Part print with two shaded views. Sizes in mm from the minimum x, y, z corner. A direction names the side the tool comes from. Coordinates: 2 decimals unless noted, no trailing zeros. Loops run counter-clockwise (first coordinate to the right, second up) from the corner with the lowest first, then second, coordinate; pieces in that order, holes last.
Item 1: Cut at B-B (y = 9.75). List the corners of the cut face in (x, z) (3 decimals), and give its area (3 significant figures).
Item 2: Cut at C-C (x = 21.75). List the corners of the cut face in (y, z), and give its area (4 significant figures).
Item 3: Drill centre lines: line 1 along Z through (x, y) = (21.75, 10.5); line 2 along X through (y, z) = (9.75, 3.25) (3 decimals); line 3 along Y through (x, z) = (27, 7.5). Where is each one in solid material? Low to high.
Item 4: Cut at D-D (x = 38.5). List the corners of the cut face in (y, z), and give its area (3 significant figures).
Item 5: Cut at A-A (z = 4.5). List the corners of the cut face in (x, y) (3 decimals).
Item 6: 3-axis set-ups, long thin cutter, end or side, ignore diameter. For the marked faces 1, 2 and 3: which of +Z, -Z, +X, -X, +Y, -Y reach the whole face in a straight line?
Item 7: Mould opens along Y. For the marked faces 4, 5 and 6 say: released by +Y, released by -Y, zero draft, split by the parting line, or undercut.
Item 8: Flat gauge pins, fed straight in: pin 1 (0.9 mm diameter, centred on y = 14, z = 8.5, fed in from -X); pin 2 (4 mm diameter, centred on x = 5, z = 5.5, fed in from -Y); pin 3 (6 mm diameter, centred on x = 32.625, y = 9.75, fed in from +Z). Where does each tip first touch, or does it go through?
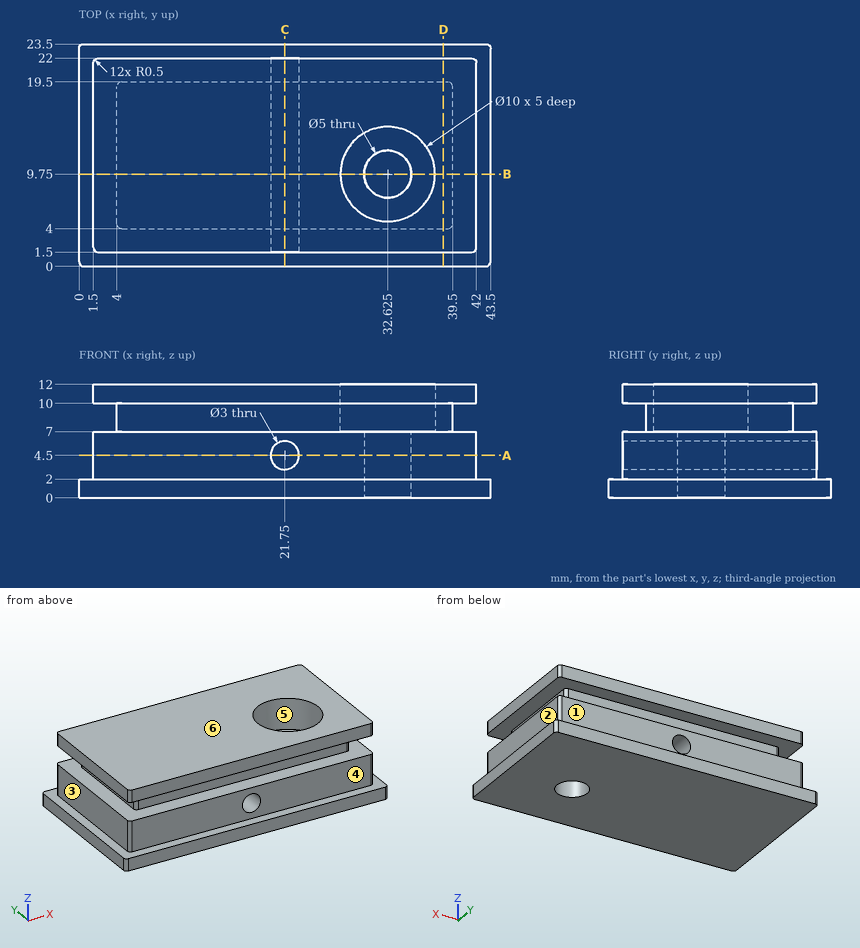
Filled sheet:
1. outline: (0, 0) - (30.125, 0) - (30.125, 7) - (27.625, 7) - (27.625, 12) - (1.5, 12) - (1.5, 10) - (4, 10) - (4, 7) - (1.5, 7) - (1.5, 2) - (0, 2) - close; (35.125, 0) - (43.5, 0) - (43.5, 2) - (42, 2) - (42, 7) - (39.5, 7) - (39.5, 10) - (42, 10) - (42, 12) - (37.625, 12) - (37.625, 7) - (35.125, 7) - close; hole circle Ø3 at (21.75, 4.5)
1. area: 385 mm2
2. outline: (0, 0) - (23.5, 0) - (23.5, 2) - (22, 2) - (22, 3) - (1.5, 3) - (1.5, 2) - (0, 2) - close; (1.5, 6) - (22, 6) - (22, 7) - (19.5, 7) - (19.5, 10) - (22, 10) - (22, 12) - (1.5, 12) - (1.5, 10) - (4, 10) - (4, 7) - (1.5, 7) - close
2. area: 175.5 mm2
3. line 1: z = 0 to 3, 6 to 12
3. line 2: x = 1.5 to 20.921, 22.579 to 30.125, 35.125 to 42
3. line 3: y = 4 to 19.5
4. outline: (0, 0) - (23.5, 0) - (23.5, 2) - (22, 2) - (22, 7) - (19.5, 7) - (19.5, 10) - (22, 10) - (22, 12) - (1.5, 12) - (1.5, 10) - (4, 10) - (4, 7) - (1.5, 7) - (1.5, 2) - (0, 2) - close
4. area: 237 mm2
5. outline: (1.5, 2) arc R0.5 ccw to (2, 1.5) - (20.25, 1.5) - (20.25, 22) - (2, 22) arc R0.5 ccw to (1.5, 21.5) - close; (23.25, 1.5) - (41.5, 1.5) arc R0.5 ccw to (42, 2) - (42, 21.5) arc R0.5 ccw to (41.5, 22) - (23.25, 22) - close; hole circle Ø5 at (32.625, 9.75)
6. face 1: +Z, +X, -X, +Y
6. face 2: +Z, +X, +Y, -Y
6. face 3: +Z, -X, +Y, -Y
7. face 4: released by -Y
7. face 5: undercut
7. face 6: zero draft
8. pin 1: stops at x = 4
8. pin 2: stops at y = 1.5
8. pin 3: stops at z = 7
